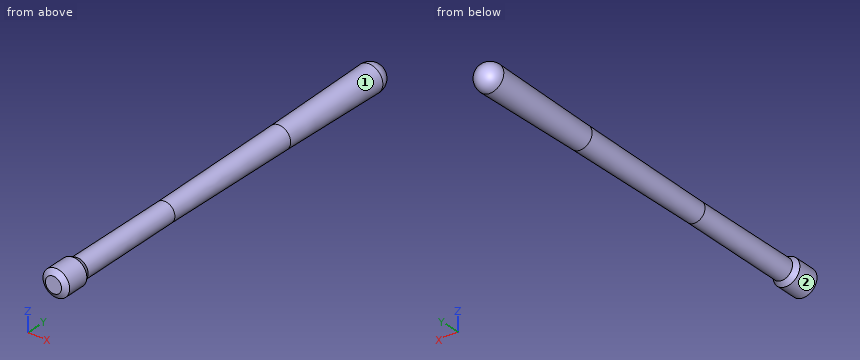
from build123d import *


with BuildPart() as part:
    # Sketch1 → Diafisis_y_cabeza (revolve)
    with BuildSketch(Plane.XY, mode=Mode.PRIVATE) as diafisis_y_cabeza_sk:
        Polygon((0, -8), (4.5, -8), (7.5, -6), (7.5, 6), (5.8, 9), (5.6, 70), (6.4, 150), (7.5, 213.424459704), (0, 213.424459704), align=None)
    revolve(diafisis_y_cabeza_sk.sketch.rotate(Axis((0, -12, 0), (0, 1, 0)), 90), axis=Axis((0, -12, 0), (0, 1, 0)))

    # Sketch2 → Extremo_proximal (revolve)
    with BuildSketch(Plane.XY):
        with BuildLine():
            Line((0, 205.924459704), (0, 220.924459704))
            ThreePointArc((0, 220.924459704), (7.5, 213.424459704), (0, 205.924459704))
        make_face()
    revolve(axis=Axis((0, 201.924459704, 0), (0, 1, 0)))


solid = part.part
For this review, take the finished solid that the model builds, in its own axes (mm). Face numbers are marked on the shaded views. Give positions to 0.01 mm unless a question says otherwise; leave off trailing zeros. Loops run counter-clockwise (first coordinate to the right, second up) from the corner with the lowest first, then second, coordinate; pieces in that order, holes last.
Item 1: Insertion check: pin 1 (3 mm diameter, centred on y = 147.5, z = -2, fed in from +X); pin 2 (5 mm diameter, centred on y = 23, z = 5, fed in from -X); pin 3 (8 mm diameter, centred on x = -2, y = 52, fed in from -Z); pin 4 (8 mm diameter, centred on x = -5.5, z = -2, fed in from -Y). Each pin has a flat end and moves straight along its axis. Give the tip position at first contact, or say it passes through.
Item 2: Take a section at A-A, the plane y = 138. State the section outline as (x, z) points.
Item 3: Draft analysis for pull direction Y (two halves, no side actions). For the marked faces 1 and 2, state which applies: +Y half, -Y half, draft (parallel to the pull), parting line (faces both ways), or undercut.
Item 4: For line 1 along X through (y, z) = (161, -2.75); line 2 along Z through (x, y) = (-1.25, 139); line 3 along Z through (x, y) = (4.25, 115), list the stretches that pass through material, from the lowest coordinate up.
Calculated:
1. pin 1: stops at x = 6.36
1. pin 2: stops at x = -5.18
1. pin 3: stops at z = -5.67
1. pin 4: stops at y = -8
2. outline: circle Ø12.56 at (0, 0)
3. face 1: undercut
3. face 2: draft
4. line 1: x = -5.99 to 5.99
4. line 2: z = -6.16 to 6.16
4. line 3: z = -4.31 to 4.31
